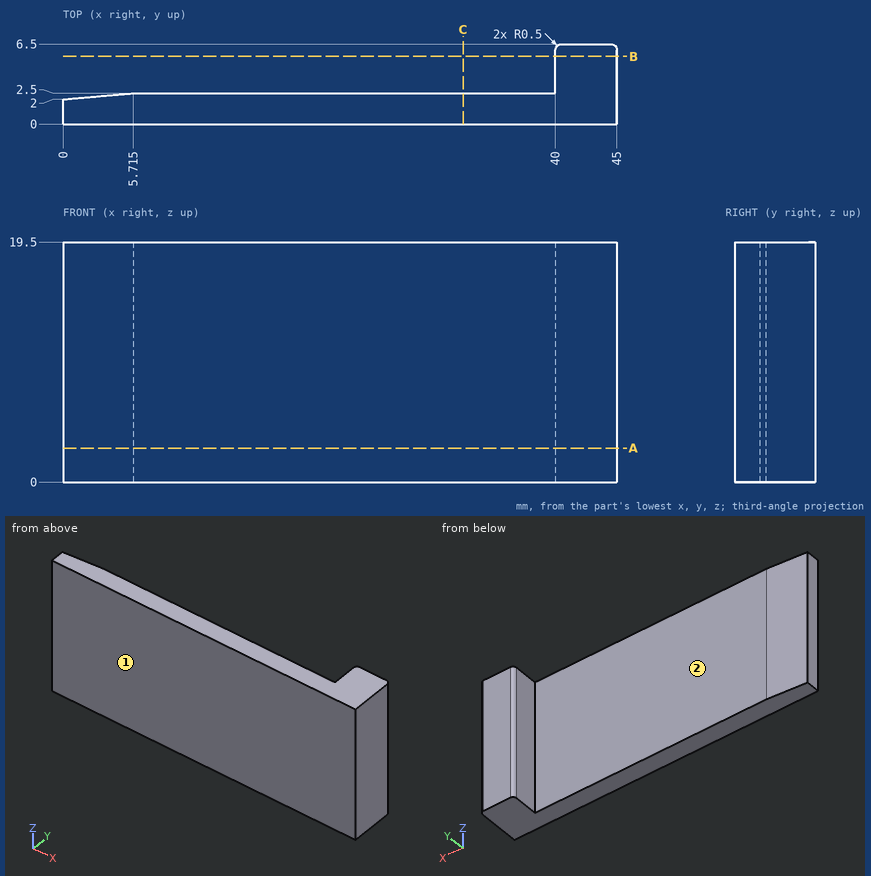
Geometry check sheet. Reference: drawing and pictorial views, mm from the part's lowest x, y, z. A direction names the side the tool comes from. Give positions to 0.01 mm unless a question says otherwise; leave off trailing zeros. Order: outer loops, then holes, each group sorted by start corner. A loop starts at its lowest first (then second) coordinate and runs counter-clockwise, first axis right, second up. Notation, with made-up numbers: M 50,32.5 L 60,32.5 A21 ccw 60,57.5 Z; hole C 26,88.25 d2. An arc over 180 degrees is marked long. Answer in a Markdown table with one row per item. Add a question column.
Q1. Sectioned sample at A-A, the plane z = 2.75. Record the boundary of the cut face in (x, y) (3 decimals).
Q2. Sectioned sample at C-C, the plane x = 32.5. Record the boundary of the cut face in (y, z).
Q3. Sectioned sample at B-B, the plane y = 5.5. Record the boundary of the cut face in (x, z).
Q4. Access from +Z, -Z, +X, -X, +Y, -Y to the whole of each face (thin tool, end or side, straight path). Record for the marked faces 1 and 2.
Q5. Thickness scan on L1, parallel to X at y = 3, z = 11.75; L2, parallel to Y at x = 39.5, z = 12.5; L3, parallel to Y at x = 5, z = 13. Record the ranges inside material, lowest first.
Q6. Gauge pin test, flat ends, axial feed: pin 1 Ø10 at (x, z) = (26, 10) entering from +Y; pin 2 Ø3 at (x, y) = (37.5, 3) entering from -Z. Record the tip position at first contact, or that the pin passes through.
Verdict:
| question | item | result |
|---|---|---|
| 1 | outline | M 0,0 L 45,0 L 45,6 A0.5 ccw 44.5,6.5 L 40.5,6.5 A0.5 ccw 40,6 L 40,2.5 L 5.715,2.5 L 0,2 Z |
| 2 | outline | M 0,0 L 2.5,0 L 2.5,19.5 L 0,19.5 Z |
| 3 | outline | M 40,0 L 45,0 L 45,19.5 L 40,19.5 Z |
| 4 | face 1 | +Z, -Z, +X, -X, -Y |
| 4 | face 2 | +Z, -Z, -X, +Y |
| 5 | L1 | 40 to 45 |
| 5 | L2 | 0 to 2.5 |
| 5 | L3 | 0 to 2.44 |
| 6 | pin 1 | y = 2.5 |
| 6 | pin 2 | z = 0 |
